Part model, mm, in its own coordinate system. A direction names the side the tool comes from. Give positions to 0.01 mm unless a question says otherwise; leave off trailing zeros. Order: outer loops, then holes, each group sorted by start corner. A loop starts at its lowest first (then second) coordinate and runs counter-clockwise, first axis right, second up.
from build123d import *

# Parameters (mm, degrees)
SKETCH_1_W          = 47
SKETCH_1_H          = 47
EXTRUDE_1_DEPTH     = 6.5
SKETCH_2_R          = 2.1
CUT_EXTRUDE_1_DEPTH = 67.785103129
SKETCH_3_W          = 34.6
SKETCH_3_H          = 34.6
CUT_EXTRUDE_2_DEPTH = 2
FILLET_1_R          = 2
FILLET_2_R          = 1.5
FILLET_3_R          = 1.5
CUT_EXTRUDE_3_DEPTH = 3.2
SKETCH_5_W          = 3.789230485
SKETCH_5_H          = 3.5
CUT_EXTRUDE_4_DEPTH = 3.2


with BuildPart() as part:
    # Эскиз1 → Бобышка-Вытянуть1 (new body)
    with BuildSketch(Plane(origin=(0, 0, 0), x_dir=(1, 0, 0), z_dir=(0, 1, 0))):
        with Locations((-23.5, 23.5)):
            Rectangle(SKETCH_1_W, SKETCH_1_H)
    extrude(amount=EXTRUDE_1_DEPTH)

    # Эскиз2 → Вырез-Вытянуть1 (cut, through all)
    with BuildSketch(Plane.XZ):
        with Locations(Location((-43.5, -3.5, 0), (0, 0, 270))):
            Circle(SKETCH_2_R)
        with Locations(Location((-3.5, -3.5, 0), (0, 0, 270))):
            Circle(SKETCH_2_R)
        with Locations(Location((-3.5, -43.5, 0), (0, 0, 270))):
            Circle(SKETCH_2_R)
        with Locations(Location((-43.5, -43.5, 0), (0, 0, 270))):
            Circle(SKETCH_2_R)
    extrude(amount=-CUT_EXTRUDE_1_DEPTH, mode=Mode.SUBTRACT)

    # Эскиз3 → Вырез-Вытянуть2 (cut)
    with BuildSketch(Plane.XZ):
        with Locations((-23.5, -23.5)):
            Rectangle(SKETCH_3_W, SKETCH_3_H)
    extrude(amount=-CUT_EXTRUDE_2_DEPTH, mode=Mode.SUBTRACT)

    # Скругление1
    fillet_1_edges = [part.edges().sort_by_distance(p)[0] for p in [
        (0, 3.25, 0),
        (-47, 3.25, 0),
        (-47, 3.25, -47),
        (0, 3.25, -47),
    ]]
    fillet(fillet_1_edges, radius=FILLET_1_R)

    # Скругление2
    fillet_2_edges = [part.edges().sort_by_distance(p)[0] for p in [
        (-40.8, 2, -23.5),
        (-23.5, 2, -6.2),
        (-6.2, 2, -23.5),
        (-23.5, 2, -40.8),
    ]]
    fillet(fillet_2_edges, radius=FILLET_2_R)

    # Скругление3
    # the kernel refuses this fillet: 1.5 mm, written as the material it adds along each edge
    with BuildSketch(Plane(origin=(-39.3, 0.5, -39.3), x_dir=(0, 0, -1), z_dir=(-1, 0, 0))) as fillet_3_piece_1_section:
        Polygon((0, 0), (FILLET_3_R, 0), (FILLET_3_R, -FILLET_3_R), (0, -FILLET_3_R), align=None)
    fillet_3_piece_1 = extrude(amount=FILLET_3_R, mode=Mode.PRIVATE)
    fillet_3_piece_1 = fillet_3_piece_1 - Plane(origin=(-39.3, 0.5, -39.3), x_dir=(0, -0.7071067811865475, 0.7071067811865475), z_dir=(-1, 0, 0)) * Sphere(FILLET_3_R, mode=Mode.PRIVATE)
    add(fillet_3_piece_1)
    with BuildSketch(Plane(origin=(-39.3, 0.5, -7.7), x_dir=(0, 0, 1), z_dir=(-1, 0, 0))) as fillet_3_piece_2_section:
        Polygon((0, 0), (FILLET_3_R, 0), (FILLET_3_R, FILLET_3_R), (0, FILLET_3_R), align=None)
    fillet_3_piece_2 = extrude(amount=FILLET_3_R, mode=Mode.PRIVATE)
    fillet_3_piece_2 = fillet_3_piece_2 - Plane(origin=(-39.3, 0.5, -7.7), x_dir=(0, -0.7071067811865475, -0.7071067811865475), z_dir=(-1, 0, 0)) * Sphere(FILLET_3_R, mode=Mode.PRIVATE)
    add(fillet_3_piece_2)
    with BuildSketch(Plane(origin=(-7.7, 0.5, -39.3), x_dir=(1, 0, 0), z_dir=(0, 0, -1))) as fillet_3_piece_3_section:
        Polygon((0, 0), (FILLET_3_R, 0), (FILLET_3_R, -FILLET_3_R), (0, -FILLET_3_R), align=None)
    fillet_3_piece_3 = extrude(amount=FILLET_3_R, mode=Mode.PRIVATE)
    fillet_3_piece_3 = fillet_3_piece_3 - Plane(origin=(-7.7, 0.5, -39.3), x_dir=(-0.7071067811865475, -0.7071067811865475, 0), z_dir=(0, 0, -1)) * Sphere(FILLET_3_R, mode=Mode.PRIVATE)
    add(fillet_3_piece_3)
    with BuildSketch(Plane(origin=(-7.7, 0.5, -7.7), x_dir=(1, 0, 0), z_dir=(0, 0, 1))) as fillet_3_piece_4_section:
        Polygon((0, 0), (FILLET_3_R, 0), (FILLET_3_R, FILLET_3_R), (0, FILLET_3_R), align=None)
    fillet_3_piece_4 = extrude(amount=FILLET_3_R, mode=Mode.PRIVATE)
    fillet_3_piece_4 = fillet_3_piece_4 - Plane(origin=(-7.7, 0.5, -7.7), x_dir=(-0.7071067811865475, -0.7071067811865475, 0), z_dir=(0, 0, 1)) * Sphere(FILLET_3_R, mode=Mode.PRIVATE)
    add(fillet_3_piece_4)
    with BuildSketch(Plane(origin=(-6.2, 0, -6.2), x_dir=(-1, 0, 0), z_dir=(0, 1, 0)), Plane(origin=(-40.8, 0, -6.2), x_dir=(0, 0, -1), z_dir=(0, 1, 0))) as fillet_3_piece_5:
        with BuildLine():
            CenterArc((FILLET_3_R, -FILLET_3_R), FILLET_3_R, 90, 90)
            Line((0, -FILLET_3_R), (0, 0))
            Line((0, 0), (FILLET_3_R, 0))
        make_face()
    extrude(amount=0.5)
    with BuildSketch(Plane(origin=(-6.2, 0, -40.8), x_dir=(-1, 0, 0), z_dir=(0, 1, 0)), Plane(origin=(-40.8, 0, -40.8), x_dir=(0, 0, 1), z_dir=(0, 1, 0))) as fillet_3_piece_6:
        with BuildLine():
            CenterArc((FILLET_3_R, FILLET_3_R), FILLET_3_R, 180, 90)
            Line((0, FILLET_3_R), (0, 0))
            Line((0, 0), (FILLET_3_R, 0))
        make_face()
    extrude(amount=0.5)

    # Эскиз4 → Вырез-Вытянуть3 (cut)
    with BuildSketch(Plane(origin=(0, 6.5, 0), x_dir=(1, 0, 0), z_dir=(0, 1, 0))):
        Polygon((-5.549593456, 39.95), (-7.599186911, 43.5), (-5.549593456, 47.05), (-1.450406544, 47.05), (0.599186911, 43.5), (-1.450406544, 39.95), align=None)
        Polygon((-39.400813089, 43.5), (-41.450406544, 47.05), (-45.549593456, 47.05), (-47.599186911, 43.5), (-45.549593456, 39.95), (-41.450406544, 39.95), align=None)
        Polygon((-1.450406544, 7.05), (-5.549593456, 7.05), (-7.599186911, 3.5), (-5.549593456, -0.05), (-1.450406544, -0.05), (0.599186911, 3.5), align=None)
        Polygon((-41.450406544, 7.05), (-39.400813089, 3.5), (-41.450406544, -0.05), (-45.549593456, -0.05), (-47.599186911, 3.5), (-45.549593456, 7.05), align=None)
    extrude(amount=-CUT_EXTRUDE_3_DEPTH, mode=Mode.SUBTRACT)

    # Эскиз5 → Вырез-Вытянуть4 (cut)
    with BuildSketch(Plane(origin=(0, 6.5, 0), x_dir=(1, 0, 0), z_dir=(0, 1, 0))):
        with Locations((-45.105384758, 45.25)):
            Rectangle(SKETCH_5_W, SKETCH_5_H)
        with Locations((-1.894615243, 45.25)):
            Rectangle(SKETCH_5_W, SKETCH_5_H)
        with Locations((-45.105384758, 1.75)):
            Rectangle(SKETCH_5_W, SKETCH_5_H)
        with Locations((-1.894615243, 1.75)):
            Rectangle(SKETCH_5_W, SKETCH_5_H)
    extrude(amount=-CUT_EXTRUDE_4_DEPTH, mode=Mode.SUBTRACT)


solid = part.part
Item 1: Band-saw the part on B-B on y = 2.75. List the corners of the cut face in (x, z), plus the area to 3 significant figures.
Item 2: Drill centre lines: probe 1 along Z at (x, y) = (-43.5, 1.6); probe 2 along Z at (x, y) = (-44, 1.5). Where is each one in solid material? Low to high.
Item 3: Band-saw the part on C-C on z = -14.5. List the corners of the cut face in (x, y), plus the area to 3 significant figures.
Item 4: Band-saw the part on D-D on x = -21. List the corners of the cut face in (y, z), plus the area to 3 significant figures.
Item 5: Band-saw the part on A-A on x = -43.5. List the corners of the cut face in (y, z), plus the area to 3 significant figures.
Item 6: Which spindle directions (+Z, -Z, +X, -X, +Y, -Y) get a long thin tool onto all of the face, cutting with end or side? Do faces 1 (the face through (-44, 5, -39.95)), 2 (the face through (-40.35, 0.25, -40.37)), 3 (the face through (-6.6, 4.92, -1.77)). Say none if no direction does.
Item 7: Drop flat-ended pins along their axis: P1, Ø1, axis at x = -3, y = 4.5, coming from the -Z side; P2, Ø2, axis at x = -45, z = -42, coming from the +Y side; P3, Ø3.5, axis at x = -4, y = 5, coming from the +Z side. Give the stop position or say it passes through.
Item 8: Pull direction Z, two halves, no side cores. Call faces 4 (the face through (-46.43, 1.67, -46.4)), 5 (the face through (-1, 3.3, -44)), 6 (the face through (-44, 5, -7.05)): released by +Z, released by -Z, zero draft, split by the parting line, or undercut.
Working result:
1. outline: (-47, -45) arc R2 ccw to (-45, -47) - (-2, -47) arc R2 ccw to (0, -45) - (0, -2) arc R2 ccw to (-2, 0) - (-45, 0) arc R2 ccw to (-47, -2) - close; hole circle Ø4.2 at (-43.5, -43.5); hole circle Ø4.2 at (-43.5, -3.5); hole circle Ø4.2 at (-3.5, -43.5); hole circle Ø4.2 at (-3.5, -3.5)
1. area: 2,150 mm2
2. probe 1: z = -47 to -45.6, -41.4 to -5.6, -1.4 to 0
2. probe 2: z = -47 to -45.54, -41.46 to -5.54, -1.46 to 0
3. outline: (-47, 0) - (-40.8, 0) - (-40.8, 0.5) arc R1.5 cw to (-39.3, 2) - (-7.7, 2) arc R1.5 cw to (-6.2, 0.5) - (-6.2, 0) - (0, 0) - (0, 6.5) - (-47, 6.5) - close
3. area: 237 mm2
4. outline: (0, -47) - (6.5, -47) - (6.5, 0) - (0, 0) - (0, -6.2) - (0.5, -6.2) arc R1.5 cw to (2, -7.7) - (2, -39.3) arc R1.5 cw to (0.5, -40.8) - (0, -40.8) - close
4. area: 237 mm2
5. outline: (0, -47) - (3.3, -47) - (3.3, -45.6) - (0, -45.6) - close; (0, -41.4) - (3.3, -41.4) - (3.3, -39.95) - (6.5, -39.95) - (6.5, -7.05) - (3.3, -7.05) - (3.3, -5.6) - (0, -5.6) - close; (0, -1.4) - (3.3, -1.4) - (3.3, 0) - (0, 0) - close
5. area: 233 mm2
6. face 1: -Z, +Y
6. face 2: -Y
6. face 3: +X, +Y
7. P1: stops at z = -39.95
7. P2: stops at y = 3.3
7. P3: stops at z = 0
8. face 4: released by -Z
8. face 5: undercut
8. face 6: released by +Z
